Autodesk Inventor part; units mm, degrees
ref_plane "YZ Plane" through (0, 0, 0) normal (1, 0, 0) x (0, 1, 0)
ref_plane "XZ Plane" through (0, 0, 0) normal (0, 1, 0) x (-1, 0, 0)
ref_plane "XY Plane" through (0, 0, 0) normal (0, 0, 1) x (1, 0, 0)
sketch "Skizze1" plane through (0, 0, 0) normal (0, 1, 0) x (-1, 0, 0)
  line L0 (-96.0755, -26.209) -> (-136.0755, -26.209)
  line L1 (-136.0755, -26.209) -> (-136.0755, -56.209)
  line L2 (-136.0755, -56.209) -> (-96.0755, -56.209)
  line L3 (-96.0755, -56.209) -> (-96.0755, -26.209)
  point P0 (0, 0)
  dimension "d0" = 40
  dimension "d1" = 30
extrude "Extrusion1" add sketch "Skizze1" along normal blind 42
sketch "Skizze2" plane through (96.0755, 0, -26.209) normal (0, 0, 1) x (1, 0, 0)
  point P0 (-96.0755, 0)
sketch "Skizze3" plane through (0, 42, 0) normal (0, 1, 0) x (1, 0, 0)
  circle A0 centre (130.0755, 50.209) radius 1.5
  circle A1 centre (111.5755, 50.209) radius 1.5
  circle A2 centre (116.0755, 31.709) radius 1.5
  line L0 (136.0755, 56.209) -> (96.0755, 56.209)
  line L1 (136.0755, 26.209) -> (136.0755, 56.209)
  point P0 (0, 0)
  dimension "d4" = 3
  dimension "d5" = 3
  dimension "d6" = 3
  dimension "d7" = 6
  dimension "d8" = 6
  dimension "d9" = 6
  dimension "d10" = 18.5
  dimension "d11" = 18.5
  dimension "d12" = 20
extrude "Extrusion2" cut sketch "Skizze3" against normal through all
properties part number "01_Coolingblock"
The model under review builds one solid part; all positions refer to its coordinate system, in mm. Coordinates: 2 decimals unless noted, no trailing zeros. Write each loop counter-clockwise with the first axis right and the second up, starting at its lowest first coordinate (ties: lowest second). Pieces come first, ordered by that corner, then holes. Notation, with made-up numbers: (72.25, 19.5) - (104.25, 19.5) arc R15 ccw to (104.25, 23.5) - close; hole circle Ø9 at (-40, -4). An arc over 180 degrees is marked (long way). Answer as CSV lines item,"result".
(1) We need section B-B (y = 10.5). Give the boundary of the cut face in (x, z), plus the area to 3 significant figures.
Data:
outline,"(96.08, -56.21) - (136.08, -56.21) - (136.08, -26.21) - (96.08, -26.21) - close; hole circle Ø3 at (111.58, -50.21); hole circle Ø3 at (116.08, -31.71); hole circle Ø3 at (130.08, -50.21)"
area,"1,180 mm2"
(2) We need section A-A (x = 130). Give the boundary of the cut face in (y, z).
Data:
outline,"(0, -56.21) - (42, -56.21) - (42, -51.71) - (0, -51.71) - close; (0, -48.71) - (42, -48.71) - (42, -26.21) - (0, -26.21) - close"
(3) For line 1 along X through (y, z) = (9, -49); line 2 along Z through (x, y) = (116, 34.5); line 3 along Z through (x, y) = (117, 36), list the stretches that pass through material, from the lowest coordinate up. Write a range as [from, to].
Data:
line 1,"x = [96.08, 110.69], [112.46, 129.19], [130.96, 136.08]"
line 2,"z = [-56.21, -33.21], [-30.21, -26.21]"
line 3,"z = [-56.21, -32.89], [-30.53, -26.21]"
